Read the model definition and answer for the solid it produces. Units are mm, in the model's axes. A direction names the side the tool comes from. Round coordinates to 2 decimals unless told otherwise and drop trailing zeros. Write each loop counter-clockwise with the first axis right and the second up, starting at its lowest first coordinate (ties: lowest second). Pieces come first, ordered by that corner, then holes. Notation, with made-up numbers: (-17, 10) - (-11, 10) arc R10 cw to (-11, 20) - close; hole circle Ø5 at (6, 47). An arc over 180 degrees is marked (long way). Answer as CSV lines item,"result". Start each with the question number.
1) Consider line 1 along Y through (x, z) = (-53.5, 7); line 2 along X through (y, z) = (-22, 1.75); line 3 along X through (y, z) = (-19.5, 3.5). Determine where each line is inside the solid, lowest interval first.
2) Which of the six approach directions +Z, -Z, +X, -X, +Y, -Y give full straight-line access (tool end or side, diameter ignored) to faces 4 (the flat face through (-64, -10, 7)), 5 (the flat face through (-62, -34, 5)), 6 (the flat face through (-46.597, -5, 2))?
3) Find section A-A on y = -20. Determine the outline of the cut face in (x, z), then the cut area to 3 significant figures.
4) Find section C-C on z = 3. Determine the outline of the cut face in (x, y).
5) Find section B-B on x = -71. Determine the outline of the cut face in (y, z).
6) Find section D-D on y = -26.5. Determine the outline of the cut face in (x, z).
7) For a pull along Y with two mould halves and no side action, classify faces 1 (the flat face through (-62, -6, 5)), 2 (the cylindrical face through (-78.508, -19.881, 2.465)), 3 (the cylindrical face through (-79.67, -32.8, 5.07)) as +Y half, -Y half, draft (parallel to the pull), parting line (faces both ways), or undercut.
8) Each of these flat-tipped pins is pushed along its axis until it touches: pin 1 (4 mm diameter, centred on x = -61.5, z = 8.5, fed in from +Y); pin 2 (4 mm diameter, centred on y = -33.5, z = 1.5, fed in from -X); pin 3 (4.5 mm diameter, centred on x = -11.1, y = -35.5, fed in from +Z). Where does it stop, or does it pass through?
from build123d import *

# Parameters (mm, degrees)
F0_W     = 34.213527
F0_H     = 20
F0_R     = 2.7
F0_R_2   = 1.7
F0_R_3   = 12
F1_DEPTH = 5
F0_H_2   = 4
F2_DEPTH = 10
F3_R     = 4


with BuildPart() as f1:
    # F0 (on Top) → F1 (new body)
    with BuildSketch(Plane.XY):
        with Locations((-63.703899, -20)):
            Rectangle(F0_W, F0_H)
        with Locations((-75.810663, -20)):
            Circle(F0_R, mode=Mode.SUBTRACT)
        with Locations((-53.597136, -20)):
            Circle(F0_R, mode=Mode.SUBTRACT)
        Polygon((-46.597136, -40), (-6.597136, -40), (-6.597136, 0), (-46.597136, 0), (-46.597136, -6), (-46.597136, -10), (-46.597136, -30), (-46.597136, -34), align=None)
        with Locations((-42.097136, -35.5)):
            Circle(F0_R_2, mode=Mode.SUBTRACT)
        with Locations((-11.097136, -35.5)):
            Circle(F0_R_2, mode=Mode.SUBTRACT)
        with Locations((-26.597136, -20)):
            Circle(F0_R_3, mode=Mode.SUBTRACT)
        with Locations((-42.097136, -4.5)):
            Circle(F0_R_2, mode=Mode.SUBTRACT)
        with Locations((-11.097136, -4.5)):
            Circle(F0_R_2, mode=Mode.SUBTRACT)
    extrude(amount=F1_DEPTH)

    # F0 (on Top) → F2 (join)
    with BuildSketch(Plane.XY):
        with Locations((-63.703899, -8)):
            Rectangle(F0_W, F0_H_2)
        with Locations((-63.703899, -32)):
            Rectangle(F0_W, F0_H_2)
    extrude(amount=F2_DEPTH)

    # F3
    f3_edges = [f1.edges().sort_by_distance(p)[0] for p in [
        (-80.810663, -6, 5),
        (-46.597136, 0, 2.5),
        (-6.597136, 0, 2.5),
        (-6.597136, -40, 2.5),
        (-46.597136, -40, 2.5),
        (-80.810663, -34, 5),
    ]]
    fillet(f3_edges, radius=F3_R)


solid = f1.part
Check values:
1,line 1,"y = -34 to -30, -10 to -6"
1,line 2,"x = -80.81 to -77.62, -74 to -55.41, -51.78 to -38.43, -14.76 to -6.6"
1,line 3,"x = -80.81 to -78.46, -73.16 to -56.25, -50.94 to -38.59, -14.61 to -6.6"
2,face 4,"+Z, +X, -X"
2,face 5,"+Z, -Z, -X, -Y"
2,face 6,"+Z, -Z, -X, +Y"
3,outline,"(-80.81, 0) - (-78.51, 0) - (-78.51, 5) - (-80.81, 5) - close; (-73.11, 0) - (-56.3, 0) - (-56.3, 5) - (-73.11, 5) - close; (-50.9, 0) - (-38.6, 0) - (-38.6, 5) - (-50.9, 5) - close; (-14.6, 0) - (-6.6, 0) - (-6.6, 5) - (-14.6, 5) - close"
3,area,"197 mm^2"
4,outline,"(-80.81, -30) arc R4 ccw to (-76.81, -34) - (-46.6, -34) - (-46.6, -36) arc R4 ccw to (-42.6, -40) - (-10.6, -40) arc R4 ccw to (-6.6, -36) - (-6.6, -4) arc R4 ccw to (-10.6, 0) - (-42.6, 0) arc R4 ccw to (-46.6, -4) - (-46.6, -6) - (-76.81, -6) arc R4 ccw to (-80.81, -10) - close; hole circle Ø5.4 at (-75.81, -20); hole circle Ø5.4 at (-53.6, -20); hole circle Ø3.4 at (-42.1, -35.5); hole circle Ø3.4 at (-42.1, -4.5); hole circle Ø24 at (-26.6, -20); hole circle Ø3.4 at (-11.1, -35.5); hole circle Ø3.4 at (-11.1, -4.5)"
5,outline,"(-34, 0) - (-6, 0) - (-6, 10) - (-10, 10) - (-10, 5) - (-30, 5) - (-30, 10) - (-34, 10) - close"
6,outline,"(-80.81, 0) - (-36.68, 0) - (-36.68, 5) - (-80.81, 5) - close; (-16.51, 0) - (-6.6, 0) - (-6.6, 5) - (-16.51, 5) - close"
7,face 1,"+Y half"
7,face 2,"undercut"
7,face 3,"-Y half"
8,pin 1,"stops at y = -6"
8,pin 2,"stops at x = -80.52"
8,pin 3,"stops at z = 5"
